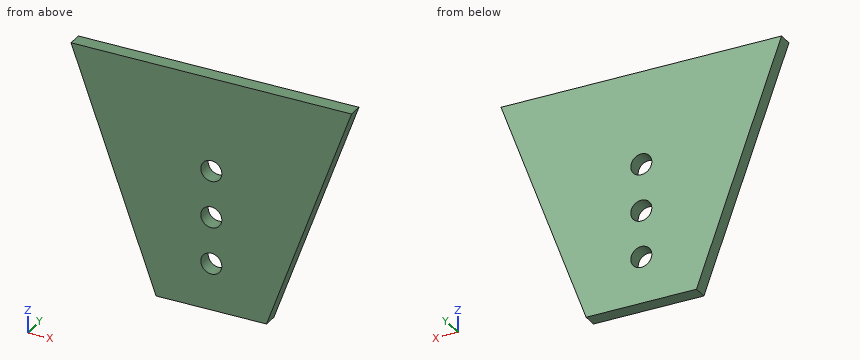
from build123d import *

# Parameters (mm, degrees)
SKETCH_1_R      = 2.25
EXTRUDE_1_DEPTH = 3


with BuildPart() as part:
    # 草图1 → 凸台-拉伸1 (new body)
    with BuildSketch(Plane(origin=(0, 0, 0), x_dir=(1, 0, 0), z_dir=(0, 1, 0))):
        Polygon((0, 0), (60, 0), (41.801488287, 50), (18.198511713, 50), align=None)
        with Locations(Location((30, 30, 0), (0, 0, 270))):
            Circle(SKETCH_1_R, mode=Mode.SUBTRACT)
        with Locations(Location((30, 20, 0), (0, 0, 270))):
            Circle(SKETCH_1_R, mode=Mode.SUBTRACT)
        with Locations(Location((30, 40, 0), (0, 0, 270))):
            Circle(SKETCH_1_R, mode=Mode.SUBTRACT)
    extrude(amount=EXTRUDE_1_DEPTH)


solid = part.part
The listing builds one solid part. Answer for the finished solid, in the listing's coordinates (mm). Round coordinates to 2 decimals unless told otherwise and drop trailing zeros. Order: outer loops, then holes, each group sorted by start corner. A loop starts at its lowest first (then second) coordinate and runs counter-clockwise, first axis right, second up. Notation, with made-up numbers: M 40,-5.5 L 90,-5.5 A14 cw 90,6.5 Z; hole C -24.5,-6 d2. An arc over 180 degrees is marked long. Answer in a Markdown table with one row per item. Add a question column.
1) The part is cut by section B-B on y = 1.55. Determine the outline of the cut face in (x, z), plus the area to 3 significant figures.
2) The part is cut by section C-C on z = -30. Determine the outline of the cut face in (x, y).
3) Consider line 1 along X through (y, z) = (0.7, -21); line 2 along X through (y, z) = (0.4, -32); line 3 along X through (y, z) = (1.95, -47.5). Determine where each line is inside the solid, lowest interval first. Write a range as from..to.
4) The part is cut by section A-A on x = 30. Determine the outline of the cut face in (y, z), plus the area to 4 significant figures.
5) Flat-ended cylindrical pins translate along their axes: pin 1 Ø1 at (y, z) = (0.5, -10.5) entering from -X; pin 2 Ø3.5 at (x, z) = (30, -40) entering from +Y; pin 3 Ø1 at (y, z) = (2, -14) entering from +X. Find the tip coordinate at first contact, or state that the pin passes through.
6) The part is cut by section D-D on z = -20. Determine the outline of the cut face in (x, y), plus the area to 3 significant figures.
Findings below:
| question | item | result |
|---|---|---|
| 1 | outline | M 0,0 L 18.2,-50 L 41.8,-50 L 60,0 Z; hole C 30,-40 d4.5; hole C 30,-30 d4.5; hole C 30,-20 d4.5 |
| 1 | area | 2,040 mm² |
| 2 | outline | M 10.92,0 L 27.75,0 L 27.75,3 L 10.92,3 Z; M 32.25,0 L 49.08,0 L 49.08,3 L 32.25,3 Z |
| 3 | line 1 | x = 7.64..27.98, 32.02..52.36 |
| 3 | line 2 | x = 11.65..28.97, 31.03..48.35 |
| 3 | line 3 | x = 17.29..42.71 |
| 4 | outline | M 0,-50 L 3,-50 L 3,-42.25 L 0,-42.25 Z; M 0,-37.75 L 3,-37.75 L 3,-32.25 L 0,-32.25 Z; M 0,-27.75 L 3,-27.75 L 3,-22.25 L 0,-22.25 Z; M 0,-17.75 L 3,-17.75 L 3,0 L 0,0 Z |
| 4 | area | 109.5 mm² |
| 5 | pin 1 | stops at x = 3.64 |
| 5 | pin 2 | passes through |
| 5 | pin 3 | stops at x = 55.09 |
| 6 | outline | M 7.28,0 L 27.75,0 L 27.75,3 L 7.28,3 Z; M 32.25,0 L 52.72,0 L 52.72,3 L 32.25,3 Z |
| 6 | area | 123 mm² |
